For this review, take the finished solid that the model builds, in its own axes (mm). A direction names the side the tool comes from. Give positions to 0.01 mm unless a question says otherwise; leave off trailing zeros. Order: outer loops, then holes, each group sorted by start corner. A loop starts at its lowest first (then second) coordinate and runs counter-clockwise, first axis right, second up.
Item 1: Consider section D-D (y = 35). Give the boundary of the cut face in (x, z).
Item 2: The part is to be moulded in two halves that separate along Z. For faces 5 (the flat face through (-19.5, 36, 19.6)), 6 (the cylindrical face through (11.923, 41.74, 3.755)), 7 (the flat face through (20, 3, -20)), say which applies: released by +Z, released by -Z, zero draft, split by the parting line, or undercut.
Item 3: For P1, Ø2.5, axis at x = -18, z = 18, coming from the +Y side; P2, Ø12, axis at x = 16.5, z = -0.5, coming from the +Y side; P3, Ø4, axis at x = 18, z = -18, coming from the +Y side, all flat-tipped, find the tip position at first contact; note any pin that passes through.
Item 4: Machinability: for faces 1 (the flat face through (19.03, 20.79, -19.09)), 2 (the cylindrical face through (1.15, 54.83, -2.22)), 3 (the flat face through (0, 60, 1.5)), 4 (the flat face through (20, 36, 19)), which of the approach directions +Z, -Z, +X, -X, +Y, -Y give a long, thin tool a straight path to every point of the face, cutting with its end or side? Answer none if there is none.
Item 5: Consider section C-C (x = 0). Give the boundary of the cut face in (y, z).
Item 6: Consider section B-B (y = 7). Give the boundary of the cut face in (x, z), plus the area to 3 significant figures.
Item 7: For probe 1 along Z at (x, y) = (18, 36.5); probe 2 along X at (y, z) = (35.5, 18), list the stretches that pass through material, from the lowest coordinate up.
Item 8: Consider section A-A (z = 0). Give the boundary of the cut face in (x, y), plus the area to 3 significant figures.
Autodesk Inventor part; units mm, degrees
ref_plane "工作平面2" through (0, 42, 0) normal (0, 1, 0) x (1, 0, 0)
ref_plane "工作平面3" through (0, 67, 0) normal (0, 1, 0) x (1, 0, 0)
ref_plane "工作平面1" through (0, 21, 0) normal (0, 1, 0) x (1, 0, 0)
sketch "草图1" plane through (0, 0, 0) normal (0, 1, 0) x (-1, 0, 0)
  line L0 (-21, 21) -> (21, 21)
  line L1 (21, 21) -> (21, -21)
  line L2 (21, -21) -> (-21, -21)
  line L3 (-21, -21) -> (-21, 21)
  line L4 (-21, 21) -> (21, -21) construction
  line L5 (21, 21) -> (-21, -21) construction
  point P0 (0, 0)
  dimension "d0" = 42
extrude "拉伸1" add sketch "草图1" along normal blind 42
sketch "草图2" plane through (0, 42, 0) normal (0, 1, 0) x (1, 0, 0)
  circle A0 centre (0, 0) radius 15
  circle A1 centre (0, 0) radius 12.5
  dimension "d3" = 30
  dimension "d4" = 25
extrude "拉伸2" cut sketch "草图2" against normal blind 1
sketch "草图3" plane through (0, 42, 0) normal (0, 1, 0) x (1, 0, 0)
  circle A0 centre (-18, -18) radius 1.5
  line L0 (0, 29.4) -> (0, -29.4) construction
  line L1 (-29.4, 0) -> (29.4, 0) construction
  circle A1 centre (18, -18) radius 1.5
  line L2 (29.4, 0) -> (-29.4, 0) construction
  circle A2 centre (-18, 18) radius 1.5
  circle A3 centre (18, 18) radius 1.5
  point P0 (0, 0)
  dimension "d8" = 3
  dimension "d9" = 18
  dimension "d10" = 18
hole "孔1" at (18, 42, 18) at (-18, 42, 18) at (-18, 42, -18) at (18, 42, -18) direction (0, -1, 0) diameter 3 depth 10 tip angle 118
thread "螺纹1"
thread "螺纹2"
thread "螺纹3"
thread "螺纹4"
ref_plane "工作平面2" through (0, 42, 0) normal (0, 1, 0) x (1, 0, 0)
sketch "草图4" plane through (0, 42, 0) normal (0, 1, 0) x (1, 0, 0)
  circle A0 centre (0, 0) radius 2.5
  dimension "d26" = 5
extrude "拉伸3" add sketch "草图4" along normal blind 25
ref_plane "工作平面3" through (0, 67, 0) normal (0, 1, 0) x (1, 0, 0)
sketch "草图5" plane through (0, 67, 0) normal (0, 1, 0) x (1, 0, 0)
  circle A0 centre (0, 0) radius 2.5
  line L0 (-2, -1.5) -> (2, -1.5)
  dimension "d29" = 1.5
extrude "拉伸4" cut sketch "草图5" against normal blind 15 contours L0 A0 picked at (-0.533956, -1.639793)
ref_plane "工作平面1" through (0, 21, 0) normal (0, 1, 0) x (1, 0, 0)
sketch "草图6" plane through (0, 21, 0) normal (0, 1, 0) x (1, 0, 0)
  circle A0 centre (-18, -18) radius 1.5
  line L0 (0, 29.4) -> (0, -29.4) construction
  line L1 (29.4, 0) -> (-29.4, 0) construction
  line L2 (-21, 21) -> (-21, -21)
  line L3 (-21, -21) -> (21, -21)
  line L4 (21, -21) -> (21, 21)
  line L5 (21, 21) -> (-21, 21)
  line L6 (-17.12132, -21) -> (-21, -17.12132)
  line L7 (-17.12132, 21) -> (-21, 17.12132)
  line L8 (17.12132, -21) -> (21, -17.12132)
  line L9 (17.12132, 21) -> (21, 17.12132)
  point P0 (0, 0)
  dimension "d34" = 45
sketch "草图6 outline for 拉伸5" plane through (0, 21, 0) normal (0, 1, 0) x (1, 0, 0)
  line L0 (-21, -17.12132) -> (-21, -21)
  line L1 (-17.12132, -21) -> (-21, -17.12132)
  line L2 (-21, -21) -> (-17.12132, -21)
extrude "拉伸5" cut sketch "草图6 outline for 拉伸5" along normal mid plane 30
mirror "镜像1" about plane through (0, 0, 0) normal (1, 0, 0) of "拉伸5"
mirror "镜像2" about plane through (0, 0, 0) normal (0, 0, 1) of "拉伸5", "镜像1"
chamfer "倒角1" distance 2 angle 45 8 edges at (21, 39, -21) (21, 3, -21) (-21, 3, -21) (-21, 39, -21) (21, 39, 21) (21, 3, 21) (-21, 39, 21) (-21, 3, 21)
sketch "草图7" plane through (0, 42, 0) normal (0, 1, 0) x (1, 0, 0)
  circle A0 centre (0, 0) radius 2.5
  circle A1 centre (0, 0) radius 12.5
extrude "拉伸6" add sketch "草图7" along normal blind 1
fillet "圆角2" radius 0.5 1 edges at (-12.5, 43, 0)
properties part number "步进电机"
Resolved:
1. outline: (-21, -17.12) - (-17.12, -21) - (17.12, -21) - (21, -17.12) - (21, 17.12) - (17.12, 21) - (-17.12, 21) - (-21, 17.12) - close; hole circle Ø3 at (-18, -18); hole circle Ø3 at (-18, 18); hole circle Ø3 at (18, -18); hole circle Ø3 at (18, 18)
2. face 5: zero draft
2. face 6: undercut
2. face 7: released by -Z
3. P1: stops at y = 31.85
3. P2: stops at y = 43
3. P3: stops at y = 42
4. face 1: -Z, +X
4. face 2: +Y
4. face 3: +Z, +X, -X, +Y
4. face 4: +Z, +X
5. outline: (0, -21) - (42, -21) - (42, -15) - (41, -15) - (41, -12.5) - (42.5, -12.5) arc R0.5 ccw to (43, -12) - (43, -2.5) - (67, -2.5) - (67, 1.5) - (52, 1.5) - (52, 2.5) - (43, 2.5) - (43, 12) arc R0.5 ccw to (42.5, 12.5) - (41, 12.5) - (41, 15) - (42, 15) - (42, 21) - (0, 21) - close
6. outline: (-21, -17.12) - (-17.12, -21) - (17.12, -21) - (21, -17.12) - (21, 17.12) - (17.12, 21) - (-17.12, 21) - (-21, 17.12) - close
6. area: 1,730 mm2
7. probe 1: z = -21 to -19.5, -16.5 to 16.5, 19.5 to 21
7. probe 2: x = -20.12 to -19.5, -16.5 to 16.5, 19.5 to 20.12
8. outline: (-21, 0) - (21, 0) - (21, 42) - (15, 42) - (15, 41) - (12.5, 41) - (12.5, 42.5) arc R0.5 ccw to (12, 43) - (2.5, 43) - (2.5, 67) - (-2.5, 67) - (-2.5, 43) - (-12, 43) arc R0.5 ccw to (-12.5, 42.5) - (-12.5, 41) - (-15, 41) - (-15, 42) - (-21, 42) - close
8. area: 1,900 mm2
